Design review of the part shown in the three views and the two pictorial views. Dimensions are in mm from the part's minimum x, y and z. Coordinates: 2 decimals unless noted, no trailing zeros. Write each loop counter-clockwise with the first axis right and the second up, starting at its lowest first coordinate (ties: lowest second). Pieces come first, ordered by that corner, then holes.
Q1. Take a section at A-A, the plane x = 13.97. Write out the cut boundary in (y, z).
Q2. The part is to be moulded in two halves that separate along Y. For the marked faces 1, 2 and 3, say which applies: released by +Y, released by -Y, zero draft, split by the parting line, or undercut.
Q3. For pin 1 Ø6 at (x, z) = (17, 33.5) entering from -Y; pin 2 Ø7.5 at (x, z) = (19, 31) entering from +Y; pin 3 Ø5 at (x, y) = (7.5, 39.5) entering from -Z, all flat-tipped, find the tip position at first contact; note any pin that passes through.
Q4. Take a section at D-D, the plane y = 14.5. Write out the cut boundary in (x, z) (1 decimal).
Q5. For L1, parallel to X at y = 67.5, z = 62.5; L2, parallel to Z at x = 13.97, y = 34; L3, parallel to Y at x = 21, z = 49.5, list the stretches that pass through material, from the lowest coordinate up.
Q6. Take a section at C-C, the plane z = 41. Write out the cut boundary in (x, y).
Q7. Take a section at B-B, the plane z = 15. Write out the cut boundary in (x, y).
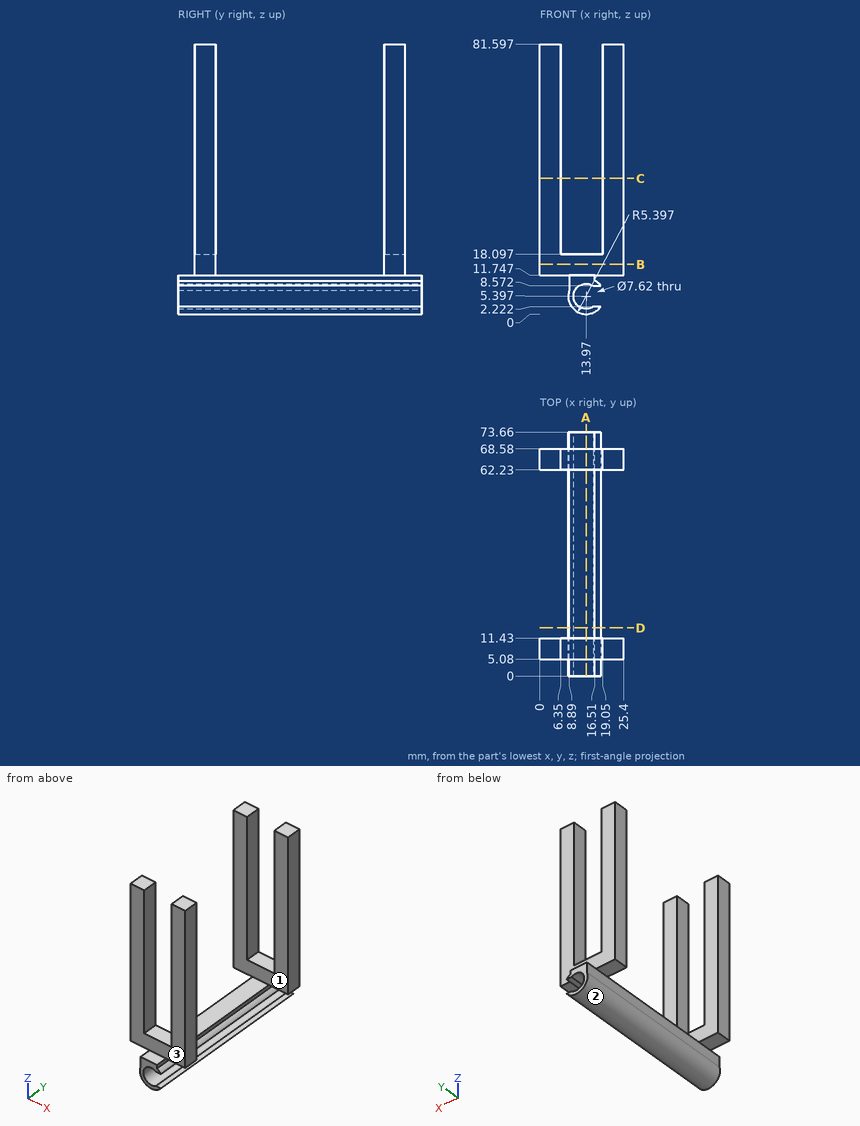
Responses:
1. outline: (0, 0) - (73.66, 0) - (73.66, 1.59) - (0, 1.59) - close; (0, 9.21) - (73.66, 9.21) - (73.66, 11.75) - (68.58, 11.75) - (68.58, 18.1) - (62.23, 18.1) - (62.23, 11.75) - (11.43, 11.75) - (11.43, 18.1) - (5.08, 18.1) - (5.08, 11.75) - (0, 11.75) - close
2. face 1: undercut
2. face 2: zero draft
2. face 3: released by -Y
3. pin 1: stops at y = 5.08
3. pin 2: stops at y = 68.58
3. pin 3: stops at z = 1.74
4. outline: (8.9, 7.2) arc R5.4 ccw to (18.3, 2.2) - (16.1, 2.2) arc R3.8 cw (long way) to (16.1, 8.6) - (18.3, 8.6) arc R5.4 ccw to (16.5, 10.2) - (16.5, 11.7) - (8.9, 11.7) - close
5. L1: x = 0 to 6.35, 19.05 to 25.4
5. L2: z = 0 to 1.59, 9.21 to 11.75
5. L3: y = 5.08 to 11.43, 62.23 to 68.58
6. outline: (0, 5.08) - (6.35, 5.08) - (6.35, 11.43) - (0, 11.43) - close; (0, 62.23) - (6.35, 62.23) - (6.35, 68.58) - (0, 68.58) - close; (19.05, 5.08) - (25.4, 5.08) - (25.4, 11.43) - (19.05, 11.43) - close; (19.05, 62.23) - (25.4, 62.23) - (25.4, 68.58) - (19.05, 68.58) - close
7. outline: (0, 5.08) - (25.4, 5.08) - (25.4, 11.43) - (0, 11.43) - close; (0, 62.23) - (25.4, 62.23) - (25.4, 68.58) - (0, 68.58) - close
